The model under review builds one solid part; all positions refer to its coordinate system, in mm. Face numbers are marked on the shaded views. A direction names the side the tool comes from. Give positions to 0.01 mm unless a question says otherwise; leave off trailing zeros. Order: outer loops, then holes, each group sorted by start corner. A loop starts at its lowest first (then second) coordinate and runs counter-clockwise, first axis right, second up.
```python
from build123d import *

# Parameters (mm, degrees)
SKETCH_2_W               = 8
SKETCH_2_H               = 5
CUT_EXTRUDE_1_DEPTH      = 0.5
SKETCH_3_W               = 8
SKETCH_3_H               = 5
CUT_EXTRUDE_2_DEPTH      = 0.5
MM_1_D                   = 3
MM_1_DEPTH               = 10
MM_1_TIP                 = 0.901290929
HOLE_WIZARD_M2_5_1_D     = 2.05
HOLE_WIZARD_M2_5_1_DEPTH = 3
HOLE_WIZARD_M2_5_1_TIP   = 0.615882135


with BuildPart() as part:
    # 草图1 → 旋转1 (revolve)
    with BuildSketch(Plane.XY, mode=Mode.PRIVATE) as revolve_1_sk:
        Polygon((0, 0), (0, 2.5), (1, 2.5), (1, 2.35), (1.6, 2.35), (1.6, 2.5), (26.5, 2.5), (26.5, 3), (31, 3), (31, 3.5), (32, 3.5), (32, 3), (39, 3), (39, 0), align=None)
    revolve(revolve_1_sk.sketch.rotate(Axis((0, 0, 0), (1, 0, 0)), 90), axis=Axis((0, 0, 0), (1, 0, 0)))

    # 草图2 → 切除-拉伸1 (cut)
    with BuildSketch(Plane.XY.offset(2.5)):
        with Locations((16, 0)):
            Rectangle(SKETCH_2_W, SKETCH_2_H)
    extrude(amount=-CUT_EXTRUDE_1_DEPTH, mode=Mode.SUBTRACT)

    # 草图3 → 切除-拉伸2 (cut)
    with BuildSketch(Plane(origin=(0, 2.5, 0), x_dir=(1, 0, 0), z_dir=(0, 1, 0))):
        with Locations((16, 0)):
            Rectangle(SKETCH_3_W, SKETCH_3_H)
    extrude(amount=-CUT_EXTRUDE_2_DEPTH, mode=Mode.SUBTRACT)

    # 大小mm 暗销孔1
    with Locations(Plane(origin=(39, 0, 0), x_dir=(0, 0, 1), z_dir=(1, 0, 0))):
        with Locations((0, 0)):
            Hole(MM_1_D / 2, depth=MM_1_DEPTH)
            with Locations((0, 0, -(MM_1_DEPTH + MM_1_TIP / 2))):  # 118° drill point
                Cone(0, MM_1_D / 2, MM_1_TIP, mode=Mode.SUBTRACT)

    # M2.5 螺纹孔1
    with Locations(Plane(origin=(35, 3, 0), x_dir=(0, 0, 1), z_dir=(0, 1, 0))):
        with Locations((0, 0)):
            Hole(HOLE_WIZARD_M2_5_1_D / 2, depth=HOLE_WIZARD_M2_5_1_DEPTH)
            with Locations((0, 0, -(HOLE_WIZARD_M2_5_1_DEPTH + HOLE_WIZARD_M2_5_1_TIP / 2))):  # 118° drill point
                Cone(0, HOLE_WIZARD_M2_5_1_D / 2, HOLE_WIZARD_M2_5_1_TIP, mode=Mode.SUBTRACT)


solid = part.part
```
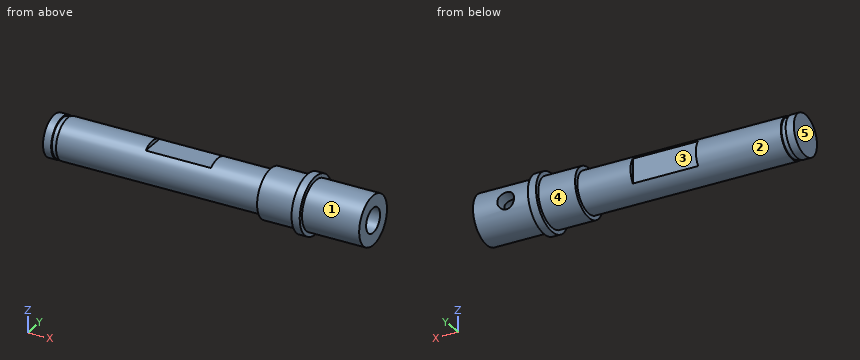
Item 1: Take a section at D-D (x = 35). Give the boundary of the cut face in (y, z) (3 decimals), and give its area (3 significant figures).
Values found:
outline: (1.095, -1.025) arc R1.5 cw (long way) to (1.095, 1.025) - (2.819, 1.025) arc R3 ccw (long way) to (2.819, -1.025) - close
area: 18.0 mm2
Item 2: Clearance check with flat-ended pins moving along their axes: pin 1 Ø3.5 at (y, z) = (0, 0.5) entering from -X; pin 2 Ø3 at (x, y) = (28.5, -1) entering from -Z; pin 3 Ø2 at (x, z) = (31, -2.5) entering from -Y; pin 4 Ø4 at (x, y) = (27, -2.5) entering from +Z. State where each tip first meets the part, or that it passes through.
Values found:
pin 1: stops at x = 0
pin 2: stops at z = -3
pin 3: stops at y = -3.16
pin 4: stops at z = 2.96
Item 3: For line 1 (Z direction, x = 35, y = 2.6) (3 decimals); line 2 (Y direction, x = 33, z = 0); line 3 (Z direction, x = 35, y = 2.2) (3 decimals), list the stretches that pass through material, from the lowest coordinate up.
Values found:
line 1: z = -1.497 to -1.025, 1.025 to 1.497
line 2: y = -3 to -1.5, 1.5 to 3
line 3: z = -2.04 to -1.025, 1.025 to 2.04
Item 4: Take a section at C-C (x = 15.5). Give the boundary of the cut face in (y, z).
Values found:
outline: (-1.5, 2) arc R2.5 ccw (long way) to (2, -1.5) - (2, 1.5) arc R2.5 ccw to (1.5, 2) - close
Item 5: Take a section at A-A (x = 30.5). Give the boundary of the cut face in (y, z).
Values found:
outline: circle Ø6 at (0, 0); hole circle Ø3 at (0, 0)
Item 6: Draft analysis for pull direction X (two halves, no side actions). For the marked faces 3, 4 and 5, state which applies: released by +X, released by -X, zero draft, split by the parting line, or undercut.
Values found:
face 3: undercut
face 4: zero draft
face 5: released by -X
Item 7: For the marked faces 1 and 2, list the 3-axis set-ups (+Z, -Z, +X, -X, +Y, -Y) from which the entire face can be reached by the end or side of a thin tool; tool diameter is ignored.
Values found:
face 1: +X
face 2: -X
Item 8: Take a section at B-B (x = 9). Give the boundary of the cut face in (y, z).
Values found:
outline: circle Ø5 at (0, 0)
